Drawing for the job (mm, zero at the part's lowest x, y, z). A direction names the side the tool comes from. Round coordinates to 2 decimals unless told otherwise and drop trailing zeros. Write each loop counter-clockwise with the first axis right and the second up, starting at its lowest first coordinate (ties: lowest second). Pieces come first, ordered by that corner, then holes. Notation, with made-up numbers: M 78,-15 L 136,-15 A27 cw 136,7 Z; hole C -18.5,-19.75 d5. An arc over 180 degrees is marked long. Use a Markdown table: item, result.
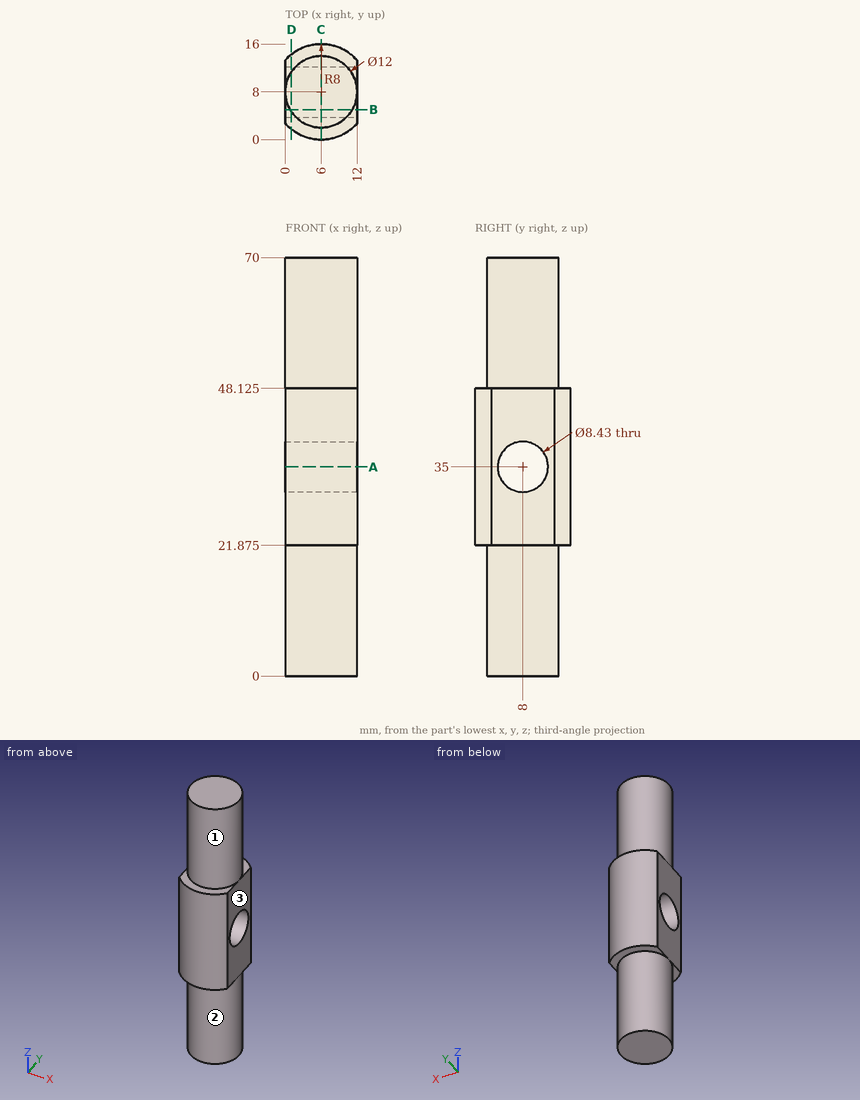
Q1. Drill centre lines: L1, parallel to Y at x = 6, z = 35 (3 decimals); L2, parallel to X at y = 7.75, z = 53; L3, parallel to Z at x = 5, y = 5. Where is each one in solid material? Low to high.
Response values:
| item | result |
|---|---|
| L1 | y = 0 to 3.785, 12.215 to 16 |
| L2 | x = 0.01 to 11.99 |
| L3 | z = 0 to 32.04, 37.96 to 70 |
Q2. Cut at C-C on x = 6. Give the cut face in (y, z) (3 decimals), and give its area (3 significant figures).
Response values:
| item | result |
|---|---|
| outline | M 0,21.875 L 2,21.875 L 2,0 L 14,0 L 14,21.875 L 16,21.875 L 16,48.125 L 14,48.125 L 14,70 L 2,70 L 2,48.125 L 0,48.125 Z; hole C 8,35 d8.43 |
| area | 889 mm2 |
Q3. Cut at B-B on y = 5. Give the cut face in (x, z) (3 decimals), and give its area (3 significant figures).
Response values:
| item | result |
|---|---|
| outline | M 0,21.875 L 0.804,21.875 L 0.804,0 L 11.196,0 L 11.196,21.875 L 12,21.875 L 12,32.039 L 0,32.039 Z; M 0,37.961 L 12,37.961 L 12,48.125 L 11.196,48.125 L 11.196,70 L 0.804,70 L 0.804,48.125 L 0,48.125 Z |
| area | 699 mm2 |
Q4. Cut at D-D on x = 1. Give the cut face in (y, z) (3 decimals), and give its area (3 significant figures).
Response values:
| item | result |
|---|---|
| outline | M 1.755,21.875 L 4.683,21.875 L 4.683,0 L 11.317,0 L 11.317,21.875 L 14.245,21.875 L 14.245,48.125 L 11.317,48.125 L 11.317,70 L 4.683,70 L 4.683,48.125 L 1.755,48.125 Z; hole C 8,35 d8.43 |
| area | 562 mm2 |
Q5. Drop flat-ended pins along their axis: P1, Ø2.5, axis at x = 7, y = 11.5, coming from the -Z side; P2, Ø2, axis at x = 9.5, z = 38, coming from the -Y side; P3, Ø1.5, axis at x = 5, z = 17, coming from the -Y side; P4, Ø5, axis at x = 2.5, z = 59, coming from the +Y side. Give the stop position or say it passes through.
Response values:
| item | result |
|---|---|
| P1 | stops at z = 0 |
| P2 | stops at y = 0.4 |
| P3 | stops at y = 2.01 |
| P4 | stops at y = 13.92 |
Q6. Cut at A-A on z = 35. Give the cut face in (x, y) (1 decimal), and give its area (3 significant figures).
Response values:
| item | result |
|---|---|
| outline | M 0,2.7 A8 ccw 12,2.7 L 12,3.8 L 0,3.8 Z; M 0,12.2 L 12,12.2 L 12,13.3 A8 ccw 0,13.3 Z |
| area | 70.9 mm2 |
Q7. Which spindle directions (+Z, -Z, +X, -X, +Y, -Y) get a long thin tool onto all of the face, cutting with end or side? Do the marked faces 1, 2 and 3. Say none if no direction does.
Response values:
| item | result |
|---|---|
| face 1 | +Z |
| face 2 | -Z |
| face 3 | +Z, -Z, +X, +Y, -Y |
